from build123d import *

# Parameters (mm, degrees)
SKETCH1_R           = 2.1463
BOSS_EXTRUDE1_DEPTH = 400
CUT_EXTRUDE1_DEPTH  = 401


with BuildPart() as part:
    # Sketch1 → Boss-Extrude1 (new body)
    with BuildSketch(Plane.XY):
        with BuildLine():
            Line((-19.9898, 7.9883), (-19.9898, 3.2893))
            ThreePointArc((-19.9898, 3.2893), (-19.75917588, 2.73252412), (-19.2024, 2.5019))
            Line((-19.2024, 2.5019), (-18.4912, 2.5019))
            ThreePointArc((-18.4912, 2.5019), (-18.275673853, 2.591173853), (-18.1864, 2.8067))
            Line((-18.1864, 2.8067), (-18.1864, 4.9149))
            ThreePointArc((-18.1864, 4.9149), (-17.668965253, 5.689295824), (-16.755503096, 5.507596904))
            Line((-16.755503096, 5.507596904), (-14.500665747, 3.252759555))
            ThreePointArc((-14.500665747, 3.252759555), (-13.850954457, 2.280397894), (-13.622806192, 1.133419111))
            Line((-13.622806192, 1.133419111), (-13.622806192, -1.133419111))
            ThreePointArc((-13.622806192, -1.133419111), (-13.850954457, -2.280397894), (-14.500665747, -3.252759555))
            Line((-14.500665747, -3.252759555), (-16.755503096, -5.507596904))
            ThreePointArc((-16.755503096, -5.507596904), (-17.668965253, -5.689295824), (-18.1864, -4.9149))
            Line((-18.1864, -4.9149), (-18.1864, -2.8067))
            ThreePointArc((-18.1864, -2.8067), (-18.275673853, -2.591173853), (-18.4912, -2.5019))
            Line((-18.4912, -2.5019), (-19.2024, -2.5019))
            ThreePointArc((-19.2024, -2.5019), (-19.75917588, -2.73252412), (-19.9898, -3.2893))
            Line((-19.9898, -3.2893), (-19.9898, -7.9883))
            ThreePointArc((-19.9898, -7.9883), (-19.402080467, -9.407180467), (-17.9832, -9.9949))
            Line((-17.9832, -9.9949), (-13.2842, -9.9949))
            ThreePointArc((-13.2842, -9.9949), (-12.72742412, -9.76427588), (-12.4968, -9.2075))
            Line((-12.4968, -9.2075), (-12.4968, -8.4963))
            ThreePointArc((-12.4968, -8.4963), (-12.586073853, -8.280773853), (-12.8016, -8.1915))
            Line((-12.8016, -8.1915), (-14.9098, -8.1915))
            ThreePointArc((-14.9098, -8.1915), (-15.684195824, -7.674065253), (-15.502496904, -6.760603096))
            Line((-15.502496904, -6.760603096), (-13.247659555, -4.505765747))
            ThreePointArc((-13.247659555, -4.505765747), (-12.275297894, -3.856054457), (-11.128319111, -3.627906192))
            Line((-11.128319111, -3.627906192), (-8.861480889, -3.627906192))
            ThreePointArc((-8.861480889, -3.627906192), (-7.714502106, -3.856054457), (-6.742140445, -4.505765747))
            Line((-6.742140445, -4.505765747), (-4.487303096, -6.760603096))
            ThreePointArc((-4.487303096, -6.760603096), (-4.305604176, -7.674065253), (-5.08, -8.1915))
            Line((-5.08, -8.1915), (-7.1882, -8.1915))
            ThreePointArc((-7.1882, -8.1915), (-7.403726147, -8.280773853), (-7.493, -8.4963))
            Line((-7.493, -8.4963), (-7.493, -9.2075))
            ThreePointArc((-7.493, -9.2075), (-7.26237588, -9.76427588), (-6.7056, -9.9949))
            Line((-6.7056, -9.9949), (0, -9.9949))
            Line((0, -9.9949), (6.7056, -9.9949))
            ThreePointArc((6.7056, -9.9949), (7.26237588, -9.76427588), (7.493, -9.2075))
            Line((7.493, -9.2075), (7.493, -8.4963))
            ThreePointArc((7.493, -8.4963), (7.403726147, -8.280773853), (7.1882, -8.1915))
            Line((7.1882, -8.1915), (5.08, -8.1915))
            ThreePointArc((5.08, -8.1915), (4.305604176, -7.674065253), (4.487303096, -6.760603096))
            Line((4.487303096, -6.760603096), (6.742140445, -4.505765747))
            ThreePointArc((6.742140445, -4.505765747), (7.714502106, -3.856054457), (8.861480889, -3.627906192))
            Line((8.861480889, -3.627906192), (11.128319111, -3.627906192))
            ThreePointArc((11.128319111, -3.627906192), (12.275297894, -3.856054457), (13.247659555, -4.505765747))
            Line((13.247659555, -4.505765747), (15.502496904, -6.760603096))
            ThreePointArc((15.502496904, -6.760603096), (15.684195824, -7.674065253), (14.9098, -8.1915))
            Line((14.9098, -8.1915), (12.8016, -8.1915))
            ThreePointArc((12.8016, -8.1915), (12.586073853, -8.280773853), (12.4968, -8.4963))
            Line((12.4968, -8.4963), (12.4968, -9.2075))
            ThreePointArc((12.4968, -9.2075), (12.72742412, -9.76427588), (13.2842, -9.9949))
            Line((13.2842, -9.9949), (17.9832, -9.9949))
            ThreePointArc((17.9832, -9.9949), (19.402080467, -9.407180467), (19.9898, -7.9883))
            Line((19.9898, -7.9883), (19.9898, -3.2893))
            ThreePointArc((19.9898, -3.2893), (19.75917588, -2.73252412), (19.2024, -2.5019))
            Line((19.2024, -2.5019), (18.4912, -2.5019))
            ThreePointArc((18.4912, -2.5019), (18.275673853, -2.591173853), (18.1864, -2.8067))
            Line((18.1864, -2.8067), (18.1864, -4.9149))
            ThreePointArc((18.1864, -4.9149), (17.668965253, -5.689295824), (16.755503096, -5.507596904))
            Line((16.755503096, -5.507596904), (14.500665747, -3.252759555))
            ThreePointArc((14.500665747, -3.252759555), (13.850954457, -2.280397894), (13.622806192, -1.133419111))
            Line((13.622806192, -1.133419111), (13.622806192, 1.133419111))
            ThreePointArc((13.622806192, 1.133419111), (13.850954457, 2.280397894), (14.500665747, 3.252759555))
            Line((14.500665747, 3.252759555), (16.755503096, 5.507596904))
            ThreePointArc((16.755503096, 5.507596904), (17.668965253, 5.689295824), (18.1864, 4.9149))
            Line((18.1864, 4.9149), (18.1864, 2.8067))
            ThreePointArc((18.1864, 2.8067), (18.275673853, 2.591173853), (18.4912, 2.5019))
            Line((18.4912, 2.5019), (19.2024, 2.5019))
            ThreePointArc((19.2024, 2.5019), (19.75917588, 2.73252412), (19.9898, 3.2893))
            Line((19.9898, 3.2893), (19.9898, 7.9883))
            ThreePointArc((19.9898, 7.9883), (19.402080467, 9.407180467), (17.9832, 9.9949))
            Line((17.9832, 9.9949), (13.2842, 9.9949))
            ThreePointArc((13.2842, 9.9949), (12.72742412, 9.76427588), (12.4968, 9.2075))
            Line((12.4968, 9.2075), (12.4968, 8.4963))
            ThreePointArc((12.4968, 8.4963), (12.586073853, 8.280773853), (12.8016, 8.1915))
            Line((12.8016, 8.1915), (14.9098, 8.1915))
            ThreePointArc((14.9098, 8.1915), (15.684195824, 7.674065253), (15.502496904, 6.760603096))
            Line((15.502496904, 6.760603096), (13.247659555, 4.505765747))
            ThreePointArc((13.247659555, 4.505765747), (12.275297894, 3.856054457), (11.128319111, 3.627906192))
            Line((11.128319111, 3.627906192), (8.861480889, 3.627906192))
            ThreePointArc((8.861480889, 3.627906192), (7.714502106, 3.856054457), (6.742140445, 4.505765747))
            Line((6.742140445, 4.505765747), (4.487303096, 6.760603096))
            ThreePointArc((4.487303096, 6.760603096), (4.305604176, 7.674065253), (5.08, 8.1915))
            Line((5.08, 8.1915), (7.1882, 8.1915))
            ThreePointArc((7.1882, 8.1915), (7.403726147, 8.280773853), (7.493, 8.4963))
            Line((7.493, 8.4963), (7.493, 9.2075))
            ThreePointArc((7.493, 9.2075), (7.26237588, 9.76427588), (6.7056, 9.9949))
            Line((6.7056, 9.9949), (0, 9.9949))
            Line((0, 9.9949), (-6.7056, 9.9949))
            ThreePointArc((-6.7056, 9.9949), (-7.26237588, 9.76427588), (-7.493, 9.2075))
            Line((-7.493, 9.2075), (-7.493, 8.4963))
            ThreePointArc((-7.493, 8.4963), (-7.403726147, 8.280773853), (-7.1882, 8.1915))
            Line((-7.1882, 8.1915), (-5.08, 8.1915))
            ThreePointArc((-5.08, 8.1915), (-4.305604176, 7.674065253), (-4.487303096, 6.760603096))
            Line((-4.487303096, 6.760603096), (-6.742140445, 4.505765747))
            ThreePointArc((-6.742140445, 4.505765747), (-7.714502106, 3.856054457), (-8.861480889, 3.627906192))
            Line((-8.861480889, 3.627906192), (-11.128319111, 3.627906192))
            ThreePointArc((-11.128319111, 3.627906192), (-12.275297894, 3.856054457), (-13.247659555, 4.505765747))
            Line((-13.247659555, 4.505765747), (-15.502496904, 6.760603096))
            ThreePointArc((-15.502496904, 6.760603096), (-15.684195824, 7.674065253), (-14.9098, 8.1915))
            Line((-14.9098, 8.1915), (-12.8016, 8.1915))
            ThreePointArc((-12.8016, 8.1915), (-12.586073853, 8.280773853), (-12.4968, 8.4963))
            Line((-12.4968, 8.4963), (-12.4968, 9.2075))
            ThreePointArc((-12.4968, 9.2075), (-12.72742412, 9.76427588), (-13.2842, 9.9949))
            Line((-13.2842, 9.9949), (-17.9832, 9.9949))
            ThreePointArc((-17.9832, 9.9949), (-19.402080467, 9.407180467), (-19.9898, 7.9883))
        make_face()
        with Locations((-9.9949, 0)):
            Circle(SKETCH1_R, mode=Mode.SUBTRACT)
        with Locations((9.9949, 0)):
            Circle(SKETCH1_R, mode=Mode.SUBTRACT)
        with BuildLine():
            Line((-6.366993808, 1.133419111), (-6.366993808, -1.133419111))
            ThreePointArc((-6.366993808, -1.133419111), (-6.138845543, -2.280397894), (-5.489134253, -3.252759555))
            Line((-5.489134253, -3.252759555), (-0.939581002, -7.802312806))
            ThreePointArc((-0.939581002, -7.802312806), (0, -8.1915), (0.939581002, -7.802312806))
            Line((0.939581002, -7.802312806), (5.489134253, -3.252759555))
            ThreePointArc((5.489134253, -3.252759555), (6.138845543, -2.280397894), (6.366993808, -1.133419111))
            Line((6.366993808, -1.133419111), (6.366993808, 1.133419111))
            ThreePointArc((6.366993808, 1.133419111), (6.138845543, 2.280397894), (5.489134253, 3.252759555))
            Line((5.489134253, 3.252759555), (0.939581002, 7.802312806))
            ThreePointArc((0.939581002, 7.802312806), (0, 8.1915), (-0.939581002, 7.802312806))
            Line((-0.939581002, 7.802312806), (-5.489134253, 3.252759555))
            ThreePointArc((-5.489134253, 3.252759555), (-6.138845543, 2.280397894), (-6.366993808, 1.133419111))
        make_face(mode=Mode.SUBTRACT)
    extrude(amount=BOSS_EXTRUDE1_DEPTH)

    # Sketch2 → Cut-Extrude1 (cut, through all)
    with BuildSketch(Plane.XY.offset(400)):
        Polygon((-20.360851008, 6.344750297), (-17.157785984, 3.141685274), (-17.157785984, -2.858314726), (-20.360851008, -6.06137975), align=None)
        Polygon((17.157785984, -2.858314726), (20.360851008, -6.06137975), (20.360851008, 6.344750297), (17.157785984, 3.141685274), align=None)
    extrude(amount=-CUT_EXTRUDE1_DEPTH, mode=Mode.SUBTRACT)


solid = part.part
Source: CAD feature listing. Evaluate the final solid. Frame: model axes, mm. Coordinates: 2 decimals unless noted, no trailing zeros. Use a Markdown table: item, result.
1) Section A-A, the plane z = 114.5. Give the number of separate pieces and of enclosed holes in the cut face, then the cut area to 3 significant figures.
Conclusion:
| item | result |
|---|---|
| separate pieces | 1 |
| enclosed holes | 3 |
| area | 312 mm^2 |
2) First-contact query: pin 1 Ø2.5 at (y, z) = (-0.5, 166.5) entering from -X; pin 2 Ø1.8 at (x, z) = (-10, 116) entering from +Y; pin 3 Ø0.5 at (y, z) = (-4.5, 221.5) entering from -X. Flat tips, straight axial feed; report the tip coordinate or a pass-through.
Conclusion:
| item | result |
|---|---|
| pin 1 | stops at x = -13.69 |
| pin 2 | stops at y = 3.63 |
| pin 3 | stops at x = -19.05 |
3) Ray query, L1, parallel to Y at x = 14.5, z = 79.5; L2, parallel to Y at x = 3, z = 154; L3, parallel to Y at x = -6.5, z = 308. Return the intervals inside material, ascending.
Conclusion:
| item | result |
|---|---|
| L1 | y = -9.99 to -8.19, -5.76 to -3.25, 3.25 to 5.76, 8.19 to 9.99 |
| L2 | y = -9.99 to -5.74, 5.74 to 9.99 |
| L3 | y = -9.99 to -8.19, -4.75 to 4.75, 8.19 to 9.99 |
4) Mould query, pull axis Y, two halves, no side actions, for faces 1 (the flat face through (0, -9.995, 197)), 2 (the flat face through (0, 9.995, 197)), 3 (the flat face through (-5, -4, 400)). Classes: pulls with the +Y half, pulls with the -Y half, needs draft (parallel to the pull), parting line crosses it, or undercut.
Conclusion:
| item | result |
|---|---|
| face 1 | pulls with the -Y half |
| face 2 | pulls with the +Y half |
| face 3 | needs draft |
